Verification items for the finished model (mm, model axes). Give positions to 0.01 mm unless a question says otherwise; leave off trailing zeros. Order: outer loops, then holes, each group sorted by start corner. A loop starts at its lowest first (then second) coordinate and runs counter-clockwise, first axis right, second up.
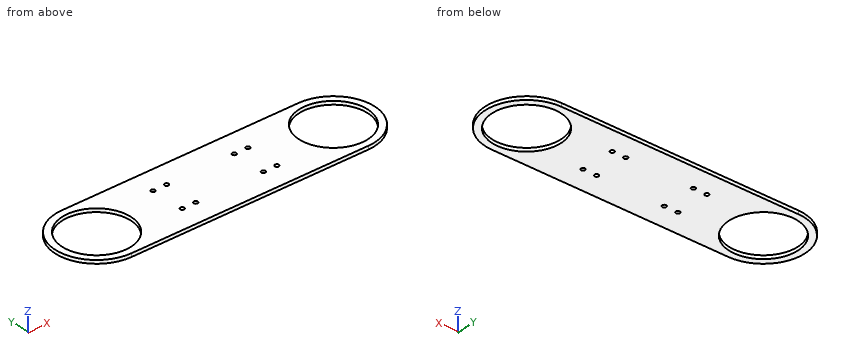
from build123d import *

# Parameters (mm, degrees)
SKETCH_2_R               = 50
SM_BASE_FLANGE_1_DEPTH   = 5
SKETCH_3_R               = 3
CUT_EXTRUDE_1_DEPTH      = 10
MIRROR_2_COPY_1_SKETCH_R = 3
MIRROR_2_COPY_1_DEPTH    = 10


# Sheet-metal steps are written as plain solids
with BuildPart() as part:
    # Sketch 2 → 基体-法兰1 (new body)
    with BuildSketch(Plane.XY):
        with BuildLine():
            Line((0, 60), (350, 60))
            ThreePointArc((350, 60), (410, 0), (350, -60))
            Line((350, -60), (0, -60))
            ThreePointArc((0, -60), (-60, 0), (0, 60))
        make_face()
        Circle(SKETCH_2_R, mode=Mode.SUBTRACT)
        with Locations((350, 0)):
            Circle(SKETCH_2_R, mode=Mode.SUBTRACT)
    extrude(amount=-SM_BASE_FLANGE_1_DEPTH)

    # 草图3 → 切除-拉伸1 (cut)
    with BuildSketch(Plane.XY):
        with Locations((225, 25)):
            Circle(SKETCH_3_R)
        with Locations((245, 25)):
            Circle(SKETCH_3_R)
    cut_extrude_1 = extrude(amount=-CUT_EXTRUDE_1_DEPTH, mode=Mode.SUBTRACT)

    # 镜向1: 切除-拉伸1 across plane
    add(cut_extrude_1.mirror(Plane.ZX), mode=Mode.SUBTRACT)

    # 镜向2: 切除-拉伸1 across plane
    add(cut_extrude_1.mirror(Plane(origin=(175, 0, 0), x_dir=(0, 0, 1), z_dir=(1, 0, 0))), mode=Mode.SUBTRACT)

    # 镜向2 copy 1 sketch → 镜向2 copy 1 (cut)
    with BuildSketch(Plane(origin=(350, 0, 0), x_dir=(-1, 0, 0), z_dir=(0, 0, 1))):
        with Locations((225, 25)):
            Circle(MIRROR_2_COPY_1_SKETCH_R)
        with Locations((245, 25)):
            Circle(MIRROR_2_COPY_1_SKETCH_R)
    extrude(amount=-MIRROR_2_COPY_1_DEPTH, mode=Mode.SUBTRACT)


solid = part.part
(1) Go/stop test with flat-tipped pins: pin 1 (5 mm diameter, centred on x = 225, y = 25, fed in from -Z); pin 2 (1 mm diameter, centred on y = 43, z = -1, fed in from +X). Record where each tip stops, or that it passes through.
Solved:
pin 1: passes through
pin 2: stops at x = 392.35
(2) Section check B-B, the plane z = -3.1. Give the number of separate pieces and of enclosed holes in the cut face, then the cut area to 3 significant figures.
Solved:
separate pieces: 1
enclosed holes: 10
area: 37,400 mm2
(3) Scan lines: line 1 (Y direction, x = 105, z = -1.5); line 2 (X direction, y = 4.5, z = -2.2); line 3 (Y direction, x = 106, z = -4.6). Record each from-to range of solid material in increasing order.
Solved:
line 1: y = -60 to -28, -22 to 22, 28 to 60
line 2: x = -59.83 to -49.8, 49.8 to 300.2, 399.8 to 409.83
line 3: y = -60 to -27.83, -22.17 to 22.17, 27.83 to 60
(4) Section check A-A, the plane x = 328.5. Enter the section's corners in (y, z), then the cut area to 3 significant figures.
Solved:
outline: (-60, -5) - (-45.14, -5) - (-45.14, 0) - (-60, 0) - close; (45.14, -5) - (60, -5) - (60, 0) - (45.14, 0) - close
area: 149 mm2
(5) Section check C-C, the plane y = -35.5. Enter the section's corners in (x, z).
Solved:
outline: (-48.37, -5) - (-35.21, -5) - (-35.21, 0) - (-48.37, 0) - close; (35.21, -5) - (314.79, -5) - (314.79, 0) - (35.21, 0) - close; (385.21, -5) - (398.37, -5) - (398.37, 0) - (385.21, 0) - close
